from build123d import *

# Parameters (mm, degrees)
F3_DEPTH = 0.5


with BuildPart() as f1:
    # F0 (on Front) → F1 (revolve)
    with BuildSketch(Plane.XZ):
        Polygon((-1.75, -1), (0, -1), (0, 10.6), (-7, 10.6), (-7, 2.1), (-2.9, 2.1), (-2.9, 0), (-1.75, 0), align=None)
    revolve(axis=Axis((0, 0, 4.8), (0, 0, -1)))

    # F2 (on face) → F3 (cut)
    with BuildSketch(Plane.XY.offset(10.6)):
        with BuildLine():
            Line((-0.5, 1.5), (0.5, 1.5))
            Line((0.5, 1.5), (0.5, 6.98212))
            ThreePointArc((0.5, 6.98212), (0, 7), (-0.5, 6.98212))
            Line((-0.5, 6.98212), (-0.5, 1.5))
        make_face()
    extrude(amount=-F3_DEPTH, mode=Mode.SUBTRACT)


solid = f1.part
Geometry: final body of the model. Coordinates: model frame, mm. A direction names the side the tool comes from. Give positions to 0.01 mm unless a question says otherwise; leave off trailing zeros. Write each loop counter-clockwise with the first axis right and the second up, starting at its lowest first coordinate (ties: lowest second). Pieces come first, ordered by that corner, then holes. Notation, with made-up numbers: (61.25, 24.25) - (116.25, 24.25) arc R22 cw to (116.25, 46.25) - close; hole circle Ø5 at (23, 45.25). An arc over 180 degrees is marked (long way). Return JSON: item names as keys, results as strings. Group by question number.
1) Section A-A on y = 0. Return the cut outline in (x, z).
2) Section B-B on x = 0. Return the cut outline in (y, z), plus the area to 3 significant figures.
3) Section D-D on y = -2.25. Return the cut outline in (x, z), plus the area to 3 significant figures.
4) First-contact query: P1, Ø3, axis at x = -3, z = 2.5, coming from the +Y side; P2, Ø5, axis at x = 5.5, z = 3, coming from the +Y side; P3, Ø5, axis at x = 0, y = -3, coming from the -Z side; P4, Ø5, axis at y = -4, z = 3, coming from the -X side. Flat tips, straight axial feed; report the tip coordinate or a pass-through.
5) Section C-C on z = 3. Return the cut outline in (x, y), plus the area to 3 significant figures.
6) Line query: line 1 (Z direction, x = 2.5, y = 3.25); line 2 (Z direction, x = -2, y = -0.5); line 3 (X direction, y = -3, z = 10.25). Output: solid intervals per line, ascending.
7) Set-up query: faces 1 (the flat face through (0, -2, 0)), 2 (the flat face through (0, 0, 10.6)), 3 (the flat face through (0, 4, 10.1)). Return all of +Z, -Z, +X, -X, +Y, -Y with unobstructed straight access to the full face (end or side cutting, diameter ignored); none if empty.
Filled in:
{
 "1": {"outline": "(-7, 2.1) - (-2.9, 2.1) - (-2.9, 0) - (-1.75, 0) - (-1.75, -1) - (1.75, -1) - (1.75, 0) - (2.9, 0) - (2.9, 2.1) - (7, 2.1) - (7, 10.6) - (-7, 10.6) - close"},
 "2": {"outline": "(-7, 2.1) - (-2.9, 2.1) - (-2.9, 0) - (-1.75, 0) - (-1.75, -1) - (1.75, -1) - (1.75, 0) - (2.9, 0) - (2.9, 2.1) - (7, 2.1) - (7, 10.1) - (1.5, 10.1) - (1.5, 10.6) - (-7, 10.6) - close", "area": "132 mm^2"},
 "3": {"outline": "(-6.63, 2.1) - (-1.83, 2.1) - (-1.83, 0) - (1.83, 0) - (1.83, 2.1) - (6.63, 2.1) - (6.63, 10.6) - (-6.63, 10.6) - close", "area": "120 mm^2"},
 "4": {"P1": "stops at y = 6.84", "P2": "stops at y = 6.32", "P3": "stops at z = -1", "P4": "stops at x = -6.84"},
 "5": {"outline": "circle Ø14 at (0, 0)", "area": "154 mm^2"},
 "6": {"line 1": "z = 2.1 to 10.6", "line 2": "z = 0 to 10.6", "line 3": "x = -6.32 to 6.32"},
 "7": {"face 1": "-Z", "face 2": "+Z, +X, -X, +Y, -Y", "face 3": "+Z, +Y"}
}
